For this review, take the finished solid that the model builds, in its own axes (mm). A direction names the side the tool comes from. Give positions to 0.01 mm unless a question says otherwise; leave off trailing zeros. Write each loop counter-clockwise with the first axis right and the second up, starting at its lowest first coordinate (ties: lowest second). Pieces come first, ordered by that corner, then holes. Notation, with made-up numbers: (63.5, 79) -> (76.5, 79) arc R28 cw to (76.5, 109) -> close; hole circle Ø6 at (72, -35). An arc over 180 degrees is marked (long way). Write item = value, one per line.
```python
from build123d import *

# Parameters (mm, degrees)
F1_DEPTH  = 4.5
F2_R      = 2.55
F3_DEPTH  = 25
F4_W      = 55
F4_H      = 8
F5_DEPTH  = 4.4
F6_R      = 2.5
F7_DEPTH  = 25
F8_R      = 2
F9_DEPTH  = 25
F10_W     = 10
F10_H     = 32
F11_DEPTH = 25
F12_R     = 4.99999
F13_R     = 4.99999
F14_R     = 2
F15_R     = 5
F16_DEPTH = 2
F18_DEPTH = 2
F19_SIZE  = 0.5
F20_SIZE  = 0.5
F21_DEPTH = 25


# Not quite as in the source:
# - a fillet or chamfer is up to 0.001 mm smaller than in the source, because OpenCascade refuses the exact size


with BuildPart() as f1:
    # F0 (on Top) → F1 (new body)
    with BuildSketch(Plane.XY):
        with BuildLine():
            Line((0, 16), (0, 0))
            Line((0, 0), (82, 0))
            Line((82, 0), (82, 68))
            Line((82, 68), (0, 68))
            Line((0, 68), (0, 52))
            Line((0, 52), (-42, 52))
            Line((-42, 52), (-42, 40))
            Line((-42, 40), (-20.0227203867, 40))
            ThreePointArc((-20.0227203867, 40), (-14.0227203867, 34), (-20.0227203867, 28))
            Line((-20.0227203867, 28), (-42, 28))
            Line((-42, 28), (-42, 16))
            Line((-42, 16), (0, 16))
        make_face()
    extrude(amount=F1_DEPTH)

    # F2 (on face) → F3 (cut)
    with BuildSketch(Plane.XY.offset(4.5)):
        with Locations((75, 57)):
            Circle(F2_R)
        with Locations((75, 11)):
            Circle(F2_R)
        with Locations((47, 57)):
            Circle(F2_R)
        with Locations((47, 11)):
            Circle(F2_R)
        with Locations((35, 57)):
            Circle(F2_R)
        with Locations((35, 11)):
            Circle(F2_R)
        with Locations((7, 57)):
            Circle(F2_R)
        with Locations((7, 11)):
            Circle(F2_R)
    extrude(amount=-F3_DEPTH, mode=Mode.SUBTRACT)

    # F4 (on face) → F5 (join)
    with BuildSketch(Plane.XY.offset(4.5)):
        with Locations((-14.5, 48)):
            Rectangle(F4_W, F4_H)
        with Locations((-14.5, 20)):
            Rectangle(F4_W, F4_H)
    extrude(amount=F5_DEPTH)

    # F6 (on face) → F7 (cut)
    with BuildSketch(Plane.XY.offset(4.5)):
        with Locations((45, 29)):
            Circle(F6_R)
        with Locations((45, 39)):
            Circle(F6_R)
    extrude(amount=-F7_DEPTH, mode=Mode.SUBTRACT)

    # F8 (on face) → F9 (cut)
    with BuildSketch(Plane(origin=(0, 0, 0), x_dir=(1, 0, 0), z_dir=(0, 0, -1))):
        with Locations((-37, -48)):
            Circle(F8_R)
        with Locations((-5, -48)):
            Circle(F8_R)
        with Locations((-37, -20)):
            Circle(F8_R)
        with Locations((-5, -20)):
            Circle(F8_R)
    extrude(amount=-F9_DEPTH, mode=Mode.SUBTRACT)

    # F10 (on face) → F11 (cut)
    with BuildSketch(Plane.XY.offset(4.5)):
        with Locations((61, 34)):
            Rectangle(F10_W, F10_H)
        with Locations((20.5358764028, 34)):
            Rectangle(F10_W, F10_H)
    extrude(amount=-F11_DEPTH, mode=Mode.SUBTRACT)

    # F12 (radius 5 in the source; OpenCascade refuses exactly that, so slightly less here)
    f12_edges = [f1.edges().sort_by_distance(p)[0] for p in [
        (15.535876, 50, 2.25),
        (25.535876, 50, 2.25),
        (15.535876, 18, 2.25),
        (25.535876, 18, 2.25),
    ]]
    fillet(f12_edges, radius=F12_R)

    # F13 (radius 5 in the source; OpenCascade refuses exactly that, so slightly less here)
    f13_edges = [f1.edges().sort_by_distance(p)[0] for p in [
        (56, 18, 2.25),
        (66, 18, 2.25),
        (66, 50, 2.25),
        (56, 50, 2.25),
    ]]
    fillet(f13_edges, radius=F13_R)

    # F14
    f14_edges = [f1.edges().sort_by_distance(p)[0] for p in [
        (13, 48, 8.9),
        (13, 20, 8.9),
    ]]
    fillet(f14_edges, radius=F14_R)

    # F15 (on face) → F16 (cut)
    with BuildSketch(Plane.XY.offset(4.5)):
        with Locations((75, 11)):
            Circle(F15_R)
        with Locations((47, 11)):
            Circle(F15_R)
        with Locations((35, 11)):
            Circle(F15_R)
        with Locations((7, 11)):
            Circle(F15_R)
        with Locations((7, 57)):
            Circle(F15_R)
        with Locations((35, 57)):
            Circle(F15_R)
        with Locations((47, 57)):
            Circle(F15_R)
        with Locations((75, 57)):
            Circle(F15_R)
    extrude(amount=-F16_DEPTH, mode=Mode.SUBTRACT)

    # F17 (on face) → F18 (cut)
    with BuildSketch(Plane(origin=(0, 0, 0), x_dir=(1, 0, 0), z_dir=(0, 0, -1))):
        with BuildLine():
            Line((40.0007831694, -39.0884933935), (40.0007694899, -38.9122828006))
            ThreePointArc((40.0007694899, -38.9122828006), (40.0000000151, -39.0003881573), (40.0007831694, -39.0884933935))
        make_face()
        with BuildLine():
            Line((40.0000000151, -29.0003881573), (40.0007694899, -38.9122828006))
            Line((40.0007694899, -38.9122828006), (40.0007831694, -39.0884933935))
            ThreePointArc((40.0007831694, -39.0884933935), (45.0442484332, -43.9998042038), (50, -38.9999999925))
            Line((50, -38.9999999925), (49.9999999849, -29.0003881573))
            ThreePointArc((49.9999999849, -29.0003881573), (45, -24), (40.0000000151, -29.0003881573))
        make_face()
    extrude(amount=-F18_DEPTH, mode=Mode.SUBTRACT)

    # F19
    f19_edges = [f1.edges().sort_by_distance(p)[0] for p in [
        (-31.01136, 28, 4.5),
        (-31.01136, 40, 4.5),
        (-14.02272, 34, 4.5),
    ]]
    chamfer(f19_edges, length=F19_SIZE)

    # F20
    f20_edges = [f1.edges().sort_by_distance(p)[0] for p in [
        (-31.01136, 40, 0),
        (-31.01136, 28, 0),
        (-14.02272, 34, 0),
    ]]
    chamfer(f20_edges, length=F20_SIZE)

    # F8 (on face) → F21 (cut)
    with BuildSketch(Plane(origin=(0, 0, 0), x_dir=(1, 0, 0), z_dir=(0, 0, -1))):
        with Locations((-37, -48)):
            Circle(F8_R)
        with Locations((-5, -48)):
            Circle(F8_R)
        with Locations((-37, -20)):
            Circle(F8_R)
        with Locations((-5, -20)):
            Circle(F8_R)
    extrude(amount=-F21_DEPTH, mode=Mode.SUBTRACT)


solid = f1.part
```
(1) Take a section at B-B (x = -5). Write out the cut boundary in (y, z), plus the area to 3 significant figures.
Answers below:
outline = (16, 0) -> (18, 0) -> (18, 8.9) -> (16, 8.9) -> close; (22, 0) -> (46, 0) -> (46, 8.9) -> (44, 8.9) -> (44, 4.5) -> (24, 4.5) -> (24, 8.9) -> (22, 8.9) -> close; (50, 0) -> (52, 0) -> (52, 8.9) -> (50, 8.9) -> close
area = 161 mm^2
(2) For pin 1 (3 mm diameter, centred on x = -33, z = 1.5, fed in from +Y); pin 2 (10 mm diameter, centred on x = 40.5, y = 32.5, fed in from +Z); pin 3 (8 mm diameter, centred on x = 75, y = 57, fed in from +Z); pin 4 (5 mm diameter, centred on x = -37, y = 48, fed in from +Z), all flat-tipped, find the tip position at first contact; note any pin that passes through.
Answers below:
pin_1 = 52
pin_2 = 4.5
pin_3 = 2.5
pin_4 = 8.9
(3) Take a section at D-D (x = 59). Write out the cut boundary in (y, z).
Answers below:
outline = (0, 0) -> (18.42, 0) -> (18.42, 4.5) -> (0, 4.5) -> close; (49.58, 0) -> (68, 0) -> (68, 4.5) -> (49.58, 4.5) -> close
(4) The part is to be moulded in two halves that separate along Y. For faces 6 (the face through (-13.889, 34.135, 0.365)), 7 (the face through (0, 60, 2)), 8 (the face through (40, 0, 2)), 9 (the face through (24.11, 48.496, 2.218)), say which applies: released by +Y, released by -Y, zero draft, split by the parting line, or undercut.
Answers below:
face_6 = undercut
face_7 = zero draft
face_8 = released by -Y
face_9 = undercut
(5) Take a section at C-C (x = 75). Write out the cut boundary in (y, z).
Answers below:
outline = (0, 0) -> (8.45, 0) -> (8.45, 2.5) -> (6, 2.5) -> (6, 4.5) -> (0, 4.5) -> close; (13.55, 0) -> (54.45, 0) -> (54.45, 2.5) -> (52, 2.5) -> (52, 4.5) -> (16, 4.5) -> (16, 2.5) -> (13.55, 2.5) -> close; (59.55, 0) -> (68, 0) -> (68, 4.5) -> (62, 4.5) -> (62, 2.5) -> (59.55, 2.5) -> close
(6) Take a section at A-A (x = -31). Write out the cut boundary in (y, z), plus the area to 3 significant figures.
Answers below:
outline = (16, 0) -> (27.5, 0) -> (28, 0.5) -> (28, 4) -> (27.5, 4.5) -> (24, 4.5) -> (24, 8.9) -> (16, 8.9) -> close; (40, 0.5) -> (40.5, 0) -> (52, 0) -> (52, 8.9) -> (44, 8.9) -> (44, 4.5) -> (40.5, 4.5) -> (40, 4) -> close
area = 178 mm^2
(7) Tool access review of faces 1 (the face through (13, 20, 6)), 2 (the face through (-15, 24, 7)), 3 (the face through (25.536, 34, 2)), 4 (the face through (45, 24, 1)), 5 (the face through (6.349, 61.957, 3.514)): name each direction out of +Z, -Z, +X, -X, +Y, -Y from which nothing blocks a thin tool from reaching the whole face with its end or side.
Answers below:
face_1 = +Z, +X, +Y, -Y
face_2 = +Z, +X, -X
face_3 = +Z, -Z
face_4 = -Z
face_5 = +Z
(8) To check wall thickness, follow probe 1 along Y at (x, z) = (75, 3.6); probe 2 along Y at (x, z) = (-16.5, 5.5); probe 3 along Y at (x, z) = (75, 0.85). State the ranges of each line that lie inside material, in increasing order.
Answers below:
probe_1 = 0 to 6, 16 to 52, 62 to 68
probe_2 = 16 to 24, 44 to 52
probe_3 = 0 to 8.45, 13.55 to 54.45, 59.55 to 68
